Input: part model. Units: mm. Frame: model coordinates. A direction names the side the tool comes from. Coordinates: 2 decimals unless noted, no trailing zeros. Write each loop counter-clockwise with the first axis right and the second up, starting at its lowest first coordinate (ties: lowest second). Pieces come first, ordered by that corner, then holes. Notation, with made-up numbers: (-40, 10) -> (2, 10) arc R22 ccw to (2, 23) -> close; hole circle Ø4 at (65, -12). An arc over 180 degrees is marked (long way). Use one line per item in the form item = value. Start each with the question number.
(1) First-contact query: pin 1 (4 mm diameter, centred on x = 18.5, z = -18.5, fed in from +Y); pin 2 (1.9 mm diameter, centred on x = 16, y = 15, fed in from -Z); pin 3 (2.5 mm diameter, centred on x = 16.5, y = -16.5, fed in from +Z); pin 4 (4.5 mm diameter, centred on x = 40, z = -3.5, fed in from +Y). Flat tips, straight axial feed; report the tip coordinate or a pass-through.
(2) Cut plane B-B on x = 15.5. Return the cut outline in (y, z) (3 decimals), plus the area to 3 significant figures.
(3) Cut plane A-A on y = 15.5. Return the cut outline in (x, z) (3 decimals), plus the area to 3 significant figures.
(4) Cut plane C-C on z = -3.5. Return the cut outline in (x, y) (3 decimals), plus the area to 3 significant figures.
(5) Set-up query: faces 5 (the face through (27.85, 14.38, -7.92)), 6 (the face through (8, 14, 4)), 7 (the face through (25, 18, -21.05)). Return all of +Z, -Z, +X, -X, +Y, -Y with unobstructed straight access to the full face (end or side cutting, diameter ignored); none if empty.
(6) Pull-direction query (Y, two-part tool) for faces 1 (the face through (-18.535, -17.827, 7.014)), 2 (the face through (9.8, 20.3, 3.9)), 3 (the face through (15, -15, 5.35)), 4 (the face through (27.85, 20.77, -17.92)); classes: released by +Y, released by -Y, zero draft, split by the parting line, or undercut.
(7) Cut plane D-D on x = 26. Return the cut outline in (y, z).
(8) Ray query, line 1 along Y through (x, z) = (15.5, 6.55) (3 decimals); line 2 along Y through (x, z) = (46.5, -24.5); line 3 along X through (y, z) = (-8.5, -21.5). Return the intervals inside material, ascending.
```python
from build123d import *

# Parameters (mm, degrees)
SKETCH1_R           = 1.85
BOSS_EXTRUDE1_DEPTH = 8
BOSS_EXTRUDE3_DEPTH = 38
CHAMFER1_SIZE       = 3.5
CHAMFER2_SIZE       = 12.5
SKETCH4_R           = 2.825
CUT_EXTRUDE1_DEPTH  = 15
CUT_EXTRUDE2_START  = -2
SKETCH5_R           = 6
CUT_EXTRUDE2_DEPTH  = 15
CHAMFER3_SIZE       = 0.5
SKETCH6_R           = 3.825
CUT_EXTRUDE3_DEPTH  = 2
SKETCH10_R          = 1.85
CUT_EXTRUDE6_DEPTH  = 10
CUT_EXTRUDE7_START  = -2.5
CUT_EXTRUDE7_DEPTH  = 2.8
SKETCH12_R          = 3.940095522
SKETCH12_R_2        = 4.765678208
PRINT_HELPER_DEPTH  = 0.65
SKETCH7_R           = 2.546325066
SKETCH7_R_2         = 2.762394701
SKETCH7_R_3         = 2.98597441
PRINT_HELPER1_DEPTH = 0.65


with BuildPart() as part:
    # Sketch1 → Boss-Extrude1 (new body)
    with BuildSketch(Plane.XY):
        with BuildLine():
            ThreePointArc((-8.94427191, -8), (8.485281374, -8.485281374), (8, 8.94427191))
            Line((8, 8.94427191), (8, 22))
            Line((8, 22), (22, 22))
            Line((22, 22), (22, -22))
            Line((22, -22), (-22, -22))
            Line((-22, -22), (-22, -8))
            Line((-22, -8), (-8.94427191, -8))
        make_face()
        with Locations((-15.5, -15.5)):
            Circle(SKETCH1_R, mode=Mode.SUBTRACT)
        with Locations((15.5, -15.5)):
            Circle(SKETCH1_R, mode=Mode.SUBTRACT)
        with Locations((15.5, 15.5)):
            Circle(SKETCH1_R, mode=Mode.SUBTRACT)
    extrude(amount=BOSS_EXTRUDE1_DEPTH)

    # Sketch3 → Boss-Extrude3 (add)
    with BuildSketch(Plane.XY.offset(8)):
        Polygon((30, -9.25), (30, -2), (50, -2), (50, 6), (30, 6), (30, 22), (22, 22), (22, 6), (22, -22), (30, -22), (30, -14.75), (34.606555482, -14.75), (34.606555482, -9.25), align=None)
    extrude(amount=-BOSS_EXTRUDE3_DEPTH)

    # Chamfer1
    chamfer1_edges = [part.edges().sort_by_distance(p)[0] for p in [
        (8, 22, 4),
        (-22, -22, 4),
        (-22, -8, 4),
    ]]
    chamfer(chamfer1_edges, length=CHAMFER1_SIZE)

    # Chamfer2
    chamfer2_edges = [part.edges().sort_by_distance(p)[0] for p in [
        (30, 6, -11),
    ]]
    chamfer(chamfer2_edges, length=CHAMFER2_SIZE)

    # Sketch4 → Cut-Extrude1 (cut)
    with BuildSketch(Plane.XZ.offset(2)):
        with Locations(Location((40, -3.5, 0), (0, 0, 270))):
            Circle(SKETCH4_R)
        with Locations(Location((40, -18.5, 0), (0, 0, 270))):
            Circle(SKETCH4_R)
    extrude(amount=-CUT_EXTRUDE1_DEPTH, mode=Mode.SUBTRACT)

    # Sketch5 → Cut-Extrude2 (cut)
    with BuildSketch(Plane(origin=(0, 6, 0), x_dir=(1, 0, 0), z_dir=(0, 1, 0)).offset(CUT_EXTRUDE2_START)):
        with Locations(Location((40, 18.5, 0), (0, 0, 65.375681648))):
            Circle(SKETCH5_R)
        with Locations(Location((40, 3.5, 0), (0, 0, 65.375681648))):
            Circle(SKETCH5_R)
    extrude(amount=CUT_EXTRUDE2_DEPTH, mode=Mode.SUBTRACT)

    # Chamfer3
    chamfer3_edges = [part.edges().sort_by_distance(p)[0] for p in [
        (22, 0, 0),
    ]]
    chamfer(chamfer3_edges, length=CHAMFER3_SIZE)

    # Sketch6 → Cut-Extrude3 (cut)
    with BuildSketch(Plane.XY.offset(8)):
        with Locations((15.5, 15.5)):
            Circle(SKETCH6_R)
        with Locations((15.5, -15.5)):
            Circle(SKETCH6_R)
        with Locations((-15.5, -15.5)):
            Circle(SKETCH6_R)
    extrude(amount=-CUT_EXTRUDE3_DEPTH, mode=Mode.SUBTRACT)

    # Sketch10 → Cut-Extrude6 (cut)
    with BuildSketch(Plane(origin=(0, 22, 0), x_dir=(1, 0, 0), z_dir=(0, 1, 0))):
        with Locations(Location((26, 8, 0), (0, 0, 180))):
            Circle(SKETCH10_R)
        with Locations(Location((26, 18, 0), (0, 0, 180))):
            Circle(SKETCH10_R)
    extrude(amount=-CUT_EXTRUDE6_DEPTH, mode=Mode.SUBTRACT)

    # Sketch11 → Cut-Extrude7 (cut)
    with BuildSketch(Plane(origin=(0, 22, 0), x_dir=(1, 0, 0), z_dir=(0, 1, 0)).offset(CUT_EXTRUDE7_START)):
        Polygon((24.239081679, 14.95), (27.760918321, 14.95), (29.521836642, 18), (27.760918321, 21.05), (24.239081679, 21.05), (20.488418147, 21.05), (20.488418147, 14.95), align=None)
        Polygon((24.239081679, 4.95), (27.760918321, 4.95), (29.521836642, 8), (27.760918321, 11.05), (24.239081679, 11.05), (20.488418147, 11.05), (20.488418147, 4.95), align=None)
    extrude(amount=-CUT_EXTRUDE7_DEPTH, mode=Mode.SUBTRACT)

    # Sketch12 → print_helper (add)
    with BuildSketch(Plane(origin=(0, 4, 0), x_dir=(1, 0, 0), z_dir=(0, 1, 0))):
        with Locations((40, 3.5)):
            Circle(SKETCH12_R)
        with Locations((40, 18.5)):
            Circle(SKETCH12_R_2)
    extrude(amount=-PRINT_HELPER_DEPTH)

    # Sketch7 → print_helper1 (add)
    with BuildSketch(Plane.XY.offset(6)):
        with Locations((15.5, 15.5)):
            Circle(SKETCH7_R)
        with Locations((15.5, -15.5)):
            Circle(SKETCH7_R_2)
        with Locations((-15.5, -15.5)):
            Circle(SKETCH7_R_3)
    extrude(amount=-PRINT_HELPER1_DEPTH)


solid = part.part
```
Values:
q1.pin_1 = through
q1.pin_2 = 5.35
q1.pin_3 = 6
q1.pin_4 = 4
q2.outline = (-22, 0) -> (-17.35, 0) -> (-17.35, 5.35) -> (-13.65, 5.35) -> (-13.65, 0) -> (13.65, 0) -> (13.65, 5.35) -> (17.35, 5.35) -> (17.35, 0) -> (22, 0) -> (22, 8) -> (19.325, 8) -> (19.325, 6) -> (11.675, 6) -> (11.675, 8) -> (-11.675, 8) -> (-11.675, 6) -> (-19.325, 6) -> (-19.325, 8) -> (-22, 8) -> close
q2.area = 282 mm2
q3.outline = (8, 0) -> (13.65, 0) -> (13.65, 5.35) -> (17.35, 5.35) -> (17.35, 0) -> (21.5, 0) -> (22, -0.5) -> (22, -30) -> (33, -30) -> (33, 8) -> (19.325, 8) -> (19.325, 6) -> (11.675, 6) -> (11.675, 8) -> (8, 8) -> close; hole circle Ø3.7 at (26, -18); hole circle Ø3.7 at (26, -8)
q3.area = 474 mm2
q4.outline = (22, -22) -> (30, -22) -> (30, -14.75) -> (34.607, -14.75) -> (34.607, -9.25) -> (30, -9.25) -> (30, -2) -> (37.175, -2) -> (37.175, 3.35) -> (42.825, 3.35) -> (42.825, -2) -> (50, -2) -> (50, 6) -> (46, 6) -> (46, 4) -> (34, 4) -> (34, 14.5) -> (30, 18.5) -> (30, 22) -> (22, 22) -> close
q4.area = 525 mm2
q5.face_5 = +Y
q5.face_6 = +Z, -Z, -X, +Y
q5.face_7 = -X
q6.face_1 = undercut
q6.face_2 = released by +Y
q6.face_3 = undercut
q6.face_4 = zero draft
q7.outline = (-22, -30) -> (22, -30) -> (22, -19.85) -> (19.5, -19.85) -> (19.5, -21.05) -> (16.7, -21.05) -> (16.7, -19.85) -> (12, -19.85) -> (12, -16.15) -> (16.7, -16.15) -> (16.7, -14.95) -> (19.5, -14.95) -> (19.5, -16.15) -> (22, -16.15) -> (22, -9.85) -> (19.5, -9.85) -> (19.5, -11.05) -> (16.7, -11.05) -> (16.7, -9.85) -> (12, -9.85) -> (12, -6.15) -> (16.7, -6.15) -> (16.7, -4.95) -> (19.5, -4.95) -> (19.5, -6.15) -> (22, -6.15) -> (22, 8) -> (-22, 8) -> close
q8.line_1 = -22 to -19.325, -11.675 to 11.675, 19.325 to 22
q8.line_2 = -2 to 6
q8.line_3 = 22 to 30
